The listing builds one solid part. Answer for the finished solid, in the listing's coordinates (mm). Face numbers are marked on the shaded views. A direction names the side the tool comes from. Round coordinates to 2 decimals unless told otherwise and drop trailing zeros. Write each loop counter-clockwise with the first axis right and the second up, starting at its lowest first coordinate (ties: lowest second). Pieces come first, ordered by that corner, then holes.
(1) A cutting plane is placed at D-D, the plane x = -3.75. Give the vertices of the cut face in (y, z).
(2) A cutting plane is placed at B-B, the plane x = 0. Give the vertices of the cut face in (y, z).
(3) Find the intervals of material crossed by probe 1 along Z at (x, y) = (-3, 0.75); probe 2 along X at (y, z) = (0, 8.2); probe 3 along X at (y, z) = (2, 5), in increasing order.
(4) A cutting plane is placed at C-C, the plane z = 5. Give the vertices of the cut face in (x, y).
(5) A cutting plane is placed at A-A, the plane y = 0. Give the vertices of the cut face in (x, z), and give its area (3 significant figures).
(6) For the marked faces 4 and 5, determine the directions among +Z, -Z, +X, -X, +Y, -Y from which every point of the face is accessible in a straight line to the end or side of a thin tool.
(7) The mould has two halves that part along X. Classify the marked faces 1, 2 and 3: +X half, -X half, draft (parallel to the pull), parting line (faces both ways), or undercut.
(8) This flat-tipped pin is pushed along its axis until it touches: pin 1 Ø2 at (x, z) = (-3, 5.5) entering from +Y. Where does it stop, or does it pass through?
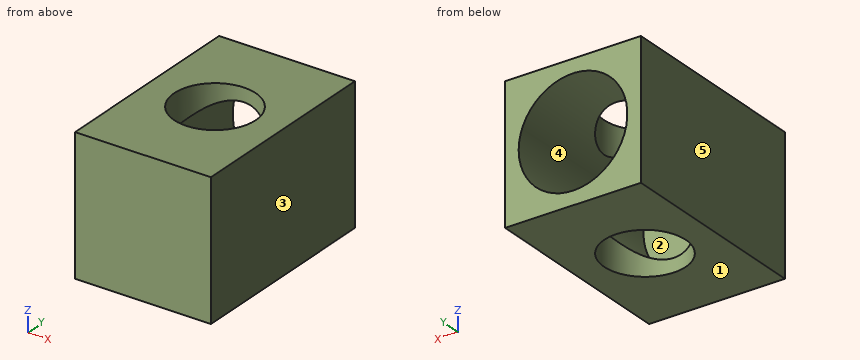
from build123d import *

# Parameters (mm, degrees)
SKETCH1_W           = 10
SKETCH1_H           = 15
SKETCH1_R           = 3
BOSS_EXTRUDE1_DEPTH = 10
SKETCH3_R           = 4
CUT_EXTRUDE1_DEPTH  = 13


with BuildPart() as part:
    # Sketch1 → Boss-Extrude1 (new body)
    with BuildSketch(Plane.XY):
        Rectangle(SKETCH1_W, SKETCH1_H)
        Circle(SKETCH1_R, mode=Mode.SUBTRACT)
    extrude(amount=BOSS_EXTRUDE1_DEPTH)

    # Sketch3 → Cut-Extrude1 (cut)
    with BuildSketch(Plane(origin=(0, 7.5, 0), x_dir=(1, 0, 0), z_dir=(0, 1, 0))):
        with Locations((0, -5)):
            Circle(SKETCH3_R)
    extrude(amount=-CUT_EXTRUDE1_DEPTH, mode=Mode.SUBTRACT)


solid = part.part
Solutions:
1. outline: (-7.5, 0) - (7.5, 0) - (7.5, 3.61) - (-5.5, 3.61) - (-5.5, 6.39) - (7.5, 6.39) - (7.5, 10) - (-7.5, 10) - close
2. outline: (-7.5, 0) - (-3, 0) - (-3, 1) - (-5.5, 1) - (-5.5, 9) - (-3, 9) - (-3, 10) - (-7.5, 10) - close; (3, 0) - (7.5, 0) - (7.5, 1) - (3, 1) - close; (3, 9) - (7.5, 9) - (7.5, 10) - (3, 10) - close
3. probe 1: z = 0 to 2.35, 7.65 to 10
3. probe 2: x = -5 to -3, 3 to 5
3. probe 3: x = -5 to -4, 4 to 5
4. outline: (-5, -7.5) - (5, -7.5) - (5, 7.5) - (4, 7.5) - (4, -5.5) - (-4, -5.5) - (-4, 7.5) - (-5, 7.5) - close
5. outline: (-5, 0) - (-3, 0) - (-3, 2.35) arc R4 cw to (-3, 7.65) - (-3, 10) - (-5, 10) - close; (3, 0) - (5, 0) - (5, 10) - (3, 10) - (3, 7.65) arc R4 cw to (3, 2.35) - close
5. area: 32.7 mm2
6. face 4: +Y
6. face 5: +Z, -Z, -X, +Y, -Y
7. face 1: draft
7. face 2: undercut
7. face 3: +X half
8. pin 1: stops at y = 7.5
